Build history of the part. All positions in model axes, mm. A direction names the side the tool comes from. Round coordinates to 2 decimals unless told otherwise and drop trailing zeros. Loops run counter-clockwise (first coordinate to the right, second up) from the corner with the lowest first, then second, coordinate; pieces in that order, holes last.
from build123d import *

# Parameters (mm, degrees)
F0_W     = 35
F0_H     = 5
F0_W_2   = 13
F0_W_3   = 5
F1_DEPTH = 63
F2_R     = 5
F3_W     = 19
F3_H     = 10
F4_DEPTH = 25
F5_SIZE  = 2
F6_R     = 2


with BuildPart() as f1:
    # F0 (on Top) → F1 (new body)
    with BuildSketch(Plane.XY):
        with Locations((-23.783123, 12.172864)):
            Rectangle(F0_W, F0_H)
        Polygon((-1.283123, 18.672864), (-6.283123, 18.672864), (-6.283123, 14.672864), (-6.283123, 9.672864), (-1.283123, 9.672864), align=None)
        with Locations((5.216877, 21.172864)):
            Rectangle(F0_W_2, F0_H)
        with Locations((-3.783123, 21.172864)):
            Rectangle(F0_W_3, F0_H)
    extrude(amount=F1_DEPTH)

    # F2
    f2_edges = [f1.edges().sort_by_distance(p)[0] for p in [
        (-41.283123, 12.172864, 63),
        (11.716877, 21.172864, 63),
        (-41.283123, 12.172864, 0),
        (11.716877, 21.172864, 0),
    ]]
    fillet(f2_edges, radius=F2_R)

    # F3 (on Front) → F4 (cut)
    with BuildSketch(Plane.XZ):
        with Locations((-23.909603, 32.153667)):
            Rectangle(F3_W, F3_H)
        with BuildLine():
            Line((-14.409603, 37.153667), (-14.409603, 27.153667))
            ThreePointArc((-14.409603, 27.153667), (-9.409603, 32.153667), (-14.409603, 37.153667))
        make_face()
        with BuildLine():
            ThreePointArc((-33.409603, 37.153667), (-38.409603, 32.153667), (-33.409603, 27.153667))
            Line((-33.409603, 27.153667), (-33.409603, 37.153667))
        make_face()
    extrude(amount=-F4_DEPTH, mode=Mode.SUBTRACT)

    # F5
    f5_edges = [f1.edges().sort_by_distance(p)[0] for p in [
        (-6.283123, 14.672864, 31.5),
    ]]
    chamfer(f5_edges, length=F5_SIZE)

    # F6
    f6_edges = [f1.edges().sort_by_distance(p)[0] for p in [
        (-6.283123, 23.672864, 31.5),
    ]]
    fillet(f6_edges, radius=F6_R)


solid = f1.part
(1) Probe line 1 (Z direction, x = -21, y = 13.5); line 2 (Y direction, x = -18, z = 25); line 3 (Y direction, x = 5, z = 17). List the from-to ranges inside material, lowest first.
Responses:
line 1: z = 0 to 27.15, 37.15 to 63
line 2: y = 9.67 to 14.67
line 3: y = 18.67 to 23.67
(2) Slice it at C-C on z = 30.5. List the corners of the cut face in (x, y), plus the area to 3 significant figures.
Responses:
outline: (-41.28, 9.67) - (-38.13, 9.67) - (-38.13, 14.67) - (-41.28, 14.67) - close; (-9.69, 9.67) - (-1.28, 9.67) - (-1.28, 18.67) - (11.72, 18.67) - (11.72, 23.67) - (-4.28, 23.67) arc R2 ccw to (-6.28, 21.67) - (-6.28, 16.67) - (-8.28, 14.67) - (-9.69, 14.67) - close
area: 169 mm2
(3) Pull direction X, two halves, no side cores. Call faces 4 (the face through (-25, 14.673, 24)), 5 (the face through (11.717, 21, 31)), 6 (the face through (-39.857, 12.208, 1.504)), 7 (the face through (-38.41, 12.14, 32.26)): +X half, -X half, draft (parallel to the pull), parting line (faces both ways), or undercut.
Responses:
face 4: draft
face 5: +X half
face 6: -X half
face 7: undercut
(4) Slice it at A-A on y = 12.25. List the corners of the cut face in (x, z), plus the area to 3 significant figures.
Responses:
outline: (-41.28, 5) arc R5 ccw to (-36.28, 0) - (-1.28, 0) - (-1.28, 63) - (-36.28, 63) arc R5 ccw to (-41.28, 58) - close; hole (-33.41, 27.15) - (-14.41, 27.15) arc R5 ccw to (-14.41, 37.15) - (-33.41, 37.15) arc R5 ccw to start
area: 2,240 mm2
(5) Slice it at B-B on x = -17.5. List the corners of the cut face in (y, z).
Responses:
outline: (9.67, 0) - (14.67, 0) - (14.67, 27.15) - (9.67, 27.15) - close; (9.67, 37.15) - (14.67, 37.15) - (14.67, 63) - (9.67, 63) - close
(6) Pin check, flat tips, straight feed: P1, Ø1, axis at x = -27, z = 11, coming from the +Y side; P2, Ø2.5, axis at y = 13.5, z = 38, coming from the +X side; P3, Ø1.5, axis at y = 19.5, z = 23, coming from the -X side. Stop position of each tip, or through.
Responses:
P1: stops at y = 14.67
P2: stops at x = -1.28
P3: stops at x = -6.28
(7) Slice it at D-D on z = 19. List the corners of the cut face in (x, y), plus the area to 3 significant figures.
Responses:
outline: (-41.28, 9.67) - (-1.28, 9.67) - (-1.28, 18.67) - (11.72, 18.67) - (11.72, 23.67) - (-4.28, 23.67) arc R2 ccw to (-6.28, 21.67) - (-6.28, 16.67) - (-8.28, 14.67) - (-41.28, 14.67) - close
area: 311 mm2
(8) Which spindle directions (+Z, -Z, +X, -X, +Y, -Y) get a long thin tool onto all of the face, cutting with end or side? Do faces 1 (the face through (5, 18.673, 31)), 2 (the face through (4, 23.673, 31)), 3 (the face through (-24, 12, 37.154)). Say none if no direction does.
Responses:
face 1: +Z, -Z, +X, -Y
face 2: +Z, -Z, +X, -X, +Y
face 3: +Y, -Y
